from build123d import *

# Parameters (mm, degrees)
SKETCH1_W                         = 458
SKETCH1_H                         = 245
BOSS_EXTRUDE1_DEPTH               = 3
CUT_EXTRUDE1_DEPTH                = 260.723410574
SKETCH3_R                         = 2.5
CUT_EXTRUDE2_DEPTH                = 260.723410574
SKETCH4_R                         = 11.5
CUT_EXTRUDE3_DEPTH                = 260.723410574
SKETCH5_W                         = 428
SKETCH5_H                         = 29
CUT_EXTRUDE4_DEPTH                = 260.723410574
SKETCH8_R                         = 1.5
SKETCH8_W                         = 69.9
SKETCH8_H                         = 41.2
CUT_EXTRUDE5_DEPTH                = 260.723410574
SKETCH9_W                         = 458
SKETCH9_H                         = 70
CUT_EXTRUDE6_DEPTH                = 10
CUT_SWITCHRUBBER_60X60_DEPTH      = 260.723410574
CUT_SWITCHRUBBER_60X60_DEPTH_BACK = 260.723410574


with BuildPart() as part:
    # Sketch1 → Boss-Extrude1 (new body)
    with BuildSketch(Plane.XY):
        Rectangle(SKETCH1_W, SKETCH1_H)
    extrude(amount=BOSS_EXTRUDE1_DEPTH)

    # Sketch2 → Cut-Extrude1 (cut, through all)
    with BuildSketch(Plane.XY.offset(3)):
        with BuildLine():
            Line((-148, -107.5), (-148, -122.5))
            ThreePointArc((-148, -122.5), (-155, -129.5), (-162, -122.5))
            Line((-162, -122.5), (-162, -107.5))
            ThreePointArc((-162, -107.5), (-155, -100.5), (-148, -107.5))
        make_face()
        with BuildLine():
            Line((162, -107.5), (162, -122.5))
            ThreePointArc((162, -122.5), (155, -129.5), (148, -122.5))
            Line((148, -122.5), (148, -107.5))
            ThreePointArc((148, -107.5), (155, -100.5), (162, -107.5))
        make_face()
    extrude(amount=-CUT_EXTRUDE1_DEPTH, mode=Mode.SUBTRACT)

    # Sketch3 → Cut-Extrude2 (cut, through all)
    with BuildSketch(Plane.XY.offset(3)):
        with Locations((-194, 112.5)):
            Circle(SKETCH3_R)
        with Locations((-194, -107.5)):
            Circle(SKETCH3_R)
        with Locations((194, -107.5)):
            Circle(SKETCH3_R)
        with Locations((194, 112.5)):
            Circle(SKETCH3_R)
        with Locations((-215, 0)):
            Circle(SKETCH3_R)
        with Locations((-215, -90)):
            Circle(SKETCH3_R)
        with Locations((-215, 90)):
            Circle(SKETCH3_R)
        with Locations((215, 0)):
            Circle(SKETCH3_R)
        with Locations((215, -90)):
            Circle(SKETCH3_R)
        with Locations((215, 90)):
            Circle(SKETCH3_R)
        with Locations((0, 112.5)):
            Circle(SKETCH3_R)
        with Locations((0, -107.5)):
            Circle(SKETCH3_R)
    extrude(amount=-CUT_EXTRUDE2_DEPTH, mode=Mode.SUBTRACT)

    # Sketch4 → Cut-Extrude3 (cut, through all)
    with BuildSketch(Plane.XY.offset(3)):
        with Locations((-39, 91)):
            Circle(SKETCH4_R)
        with Locations((39, 91)):
            Circle(SKETCH4_R)
    extrude(amount=-CUT_EXTRUDE3_DEPTH, mode=Mode.SUBTRACT)

    # Sketch5 → Cut-Extrude4 (cut, through all)
    with BuildSketch(Plane.XY.offset(3)):
        with Locations((0, 53)):
            Rectangle(SKETCH5_W, SKETCH5_H)
    extrude(amount=-CUT_EXTRUDE4_DEPTH, mode=Mode.SUBTRACT)

    # Sketch8 → Cut-Extrude5 (cut, through all)
    with BuildSketch(Plane.XY.offset(3)):
        with Locations((5.296172264, 15.703565509)):
            Circle(SKETCH8_R)
        with Locations((5.679687501, -26.054673392)):
            Circle(SKETCH8_R)
        with Locations((-83.3, 14.88)):
            Circle(SKETCH8_R)
        with Locations((-83.367997673, -26.737946691)):
            Circle(SKETCH8_R)
        with Locations((-39, -5.5)):
            Rectangle(SKETCH8_W, SKETCH8_H)
    extrude(amount=-CUT_EXTRUDE5_DEPTH, mode=Mode.SUBTRACT)

    # Sketch9 → Cut-Extrude6 (cut)
    with BuildSketch(Plane.XY.offset(3)):
        with Locations((0, 87.5)):
            Rectangle(SKETCH9_W, SKETCH9_H)
    extrude(amount=-CUT_EXTRUDE6_DEPTH, mode=Mode.SUBTRACT)

    # Sketch11 → Cut_SwitchRubber_60x60 (cut, two sides: drawn at the far end of the back side and taken through both)
    with BuildSketch(Plane.XY.offset(-CUT_SWITCHRUBBER_60X60_DEPTH_BACK)):
        with BuildLine():
            Line((99.5, -27), (149.5, -27))
            ThreePointArc((149.5, -27), (153.035533906, -25.535533906), (154.5, -22))
            Line((154.5, -22), (154.5, 28))
            ThreePointArc((154.5, 28), (153.035533906, 31.535533906), (149.5, 33))
            Line((149.5, 33), (99.5, 33))
            ThreePointArc((99.5, 33), (95.964466094, 31.535533906), (94.5, 28))
            Line((94.5, 28), (94.5, -22))
            ThreePointArc((94.5, -22), (95.964466094, -25.535533906), (99.5, -27))
        make_face()
    extrude(amount=CUT_SWITCHRUBBER_60X60_DEPTH + CUT_SWITCHRUBBER_60X60_DEPTH_BACK, mode=Mode.SUBTRACT)


solid = part.part
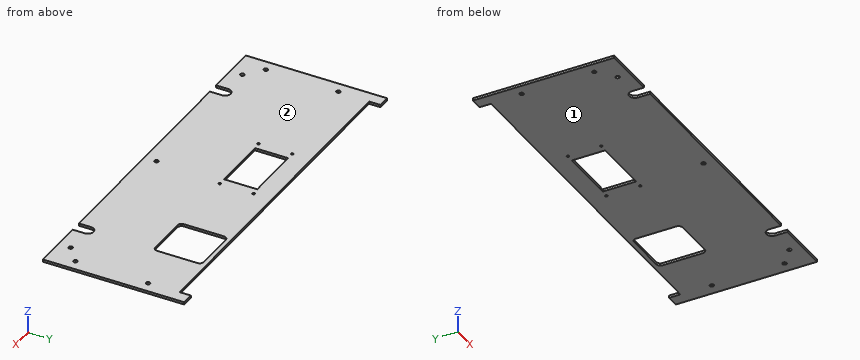
Geometry check sheet. Reference: the model listing, model coordinates, mm. Face numbers are marked on the shaded views. Give positions to 0.01 mm unless a question says otherwise; leave off trailing zeros. Loops run counter-clockwise (first coordinate to the right, second up) from the corner with the lowest first, then second, coordinate; pieces in that order, holes last.
(1) Section check C-C on x = -187. Record the cut outline in (y, z).
From the geometry:
outline: (-122.5, 0) - (38.5, 0) - (38.5, 3) - (-122.5, 3) - close
(2) Depth check by flat-ended pin: pin 1 Ø1.8 at (x, y) = (-83.37, -26.74) entering from +Z; pin 2 Ø1.5 at (x, y) = (68.5, 15) entering from -Z; pin 3 Ø1.5 at (x, z) = (119, 1) entering from +Y. Enter the tip coordinate at first touch or a pass-through.
From the geometry:
pin 1: passes through
pin 2: stops at z = 0
pin 3: stops at y = 38.5
(3) Section check A-A on x = 120.5. Record the cut outline in (y, z).
From the geometry:
outline: (-122.5, 0) - (-27, 0) - (-27, 3) - (-122.5, 3) - close; (33, 0) - (38.5, 0) - (38.5, 3) - (33, 3) - close
(4) Section check B-B on x = -65.5. Record the cut outline in (y, z), then the cut area to 3 significant figures.
From the geometry:
outline: (-122.5, 0) - (-26.1, 0) - (-26.1, 3) - (-122.5, 3) - close; (15.1, 0) - (38.5, 0) - (38.5, 3) - (15.1, 3) - close
area: 359 mm2
(5) Section check D-D on z = 1.1. Count the separate pieces of the cut face and the enclosed holes in it, then the cut area to 3 significant figures.
From the geometry:
separate pieces: 1
enclosed holes: 13
area: 67,000 mm2
(6) Thickness scan on L1, parallel to Y at x = -215, z = 1.7; L2, parallel to X at y = -112.5, z = 2.5; L3, parallel to X at y = -7, z = 1.1. Record the ranges inside material, lowest first.
From the geometry:
L1: y = -122.5 to -92.5, -87.5 to -2.5, 2.5 to 52.5
L2: x = -229 to -162, -148 to 148, 162 to 229
L3: x = -229 to -73.95, -4.05 to 94.5, 154.5 to 229
(7) Release check for a two-part mould opening along Z. For the marked faces 1 and 2 record: released by +Z, released by -Z, zero draft, split by the parting line, or undercut.
From the geometry:
face 1: released by -Z
face 2: released by +Z
